The figure shows three views and two pictorial views of one solid part (mm, origin at its lowest corner). Answer the questions. Round coordinates to 2 decimals unless told otherwise and drop trailing zeros. Write each loop counter-clockwise with the first axis right and the second up, starting at its lowest first coordinate (ties: lowest second). Pieces come first, ordered by that corner, then holes. Notation, with made-up numbers: M 66.5,39 L 117.5,39 A25 cw 117.5,59 Z; hole C -29.5,16.5 d9. An arc over 180 degrees is marked long. One line per item, written item: value. Start each with the question number.
Q1. Find section D-D (y = 55.5). Write down the section's boundary in (x, z).
Q2. Find section C-C (x = 21). Write down the section's boundary in (y, z), and give its area (3 significant figures).
Q3. Find section B-B (z = 2.5). Write down the section's boundary in (x, y), and give its area (3 significant figures).
Q4. Consider probe 1 along X at (y, z) = (62, 6.75); probe 2 along X at (y, z) = (48, 0.75); probe 3 along Z at (x, y) = (64.7, 39.5). Determine where each line is inside the solid, lowest interval first.
Q5. Given pin 1 Ø20 at (x, y) = (33.5, 40) entering from -Z; pin 2 Ø1.6 at (x, z) = (1, 2) entering from -Y; pin 3 Ø1.5 at (y, z) = (27, 2.5) entering from +X, each flat-ended and moving along its own axis, determine where each tip first touches the part or whether it passes through.
Q6. The mould has two halves that part along X. Classify the marked faces 1 and 2: released by +X, released by -X, zero draft, split by the parting line, or undercut.
Q7. Find section A-A (y = 39.5). Write down the section's boundary in (x, z), and give its area (3 significant figures).
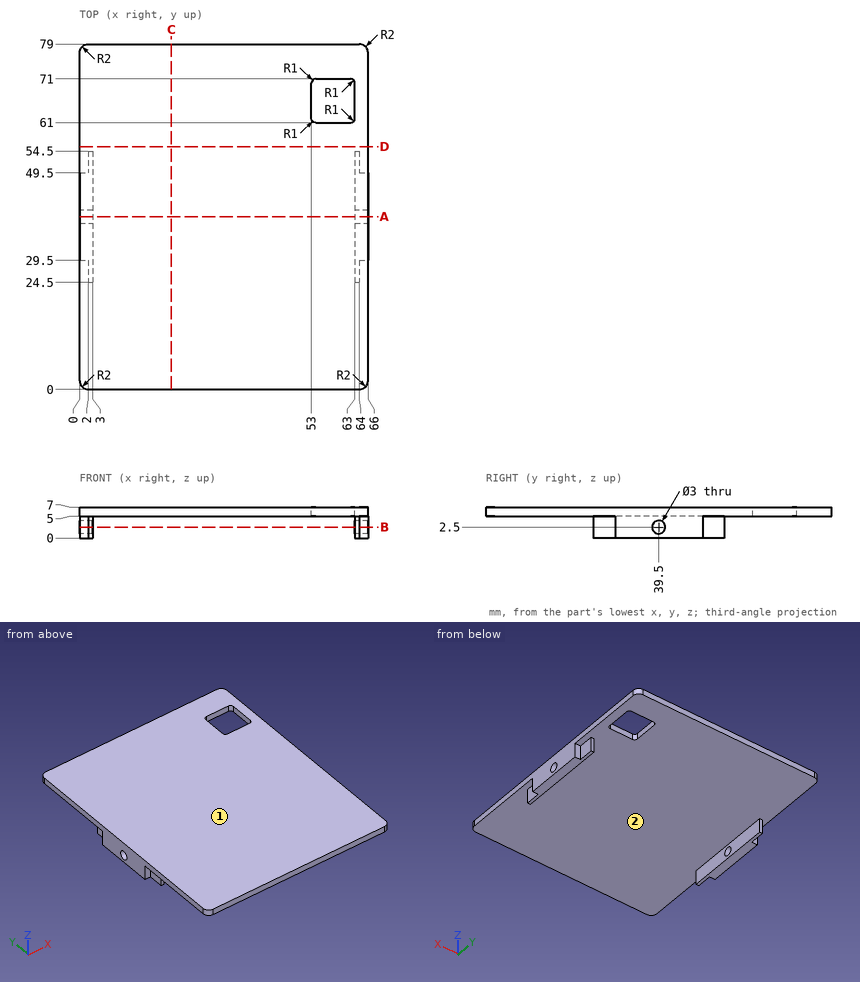
The answers:
1. outline: M 0,5 L 66,5 L 66,7 L 0,7 Z
2. outline: M 0,5 L 79,5 L 79,7 L 0,7 Z
2. area: 158 mm2
3. outline: M 0,29.5 L 2,29.5 L 2,24.5 L 3,24.5 L 3,38 L 0,38 Z; M 0,41 L 3,41 L 3,54.5 L 2,54.5 L 2,49.5 L 0,49.5 Z; M 63,24.5 L 64,24.5 L 64,29.5 L 66,29.5 L 66,38 L 63,38 Z; M 63,41 L 66,41 L 66,49.5 L 64,49.5 L 64,54.5 L 63,54.5 Z
3. area: 122 mm2
4. probe 1: 0 to 53, 63 to 66
4. probe 2: 0 to 3, 63 to 66
4. probe 3: 0 to 1, 4 to 7
5. pin 1: z = 5
5. pin 2: y = 29.5
5. pin 3: x = 64
6. face 1: zero draft
6. face 2: undercut
7. outline: M 0,0 L 3,0 L 3,1 L 0,1 Z; M 0,4 L 3,4 L 3,5 L 63,5 L 63,4 L 66,4 L 66,7 L 0,7 Z; M 63,0 L 66,0 L 66,1 L 63,1 Z
7. area: 144 mm2
